Design review of the part shown in the three views and the two pictorial views. Dimensions are in mm from the part's minimum x, y and z. A direction names the side the tool comes from. Give positions to 0.01 mm unless a question says otherwise; leave off trailing zeros. Loops run counter-clockwise (first coordinate to the right, second up) from the corner with the lowest first, then second, coordinate; pieces in that order, holes last.
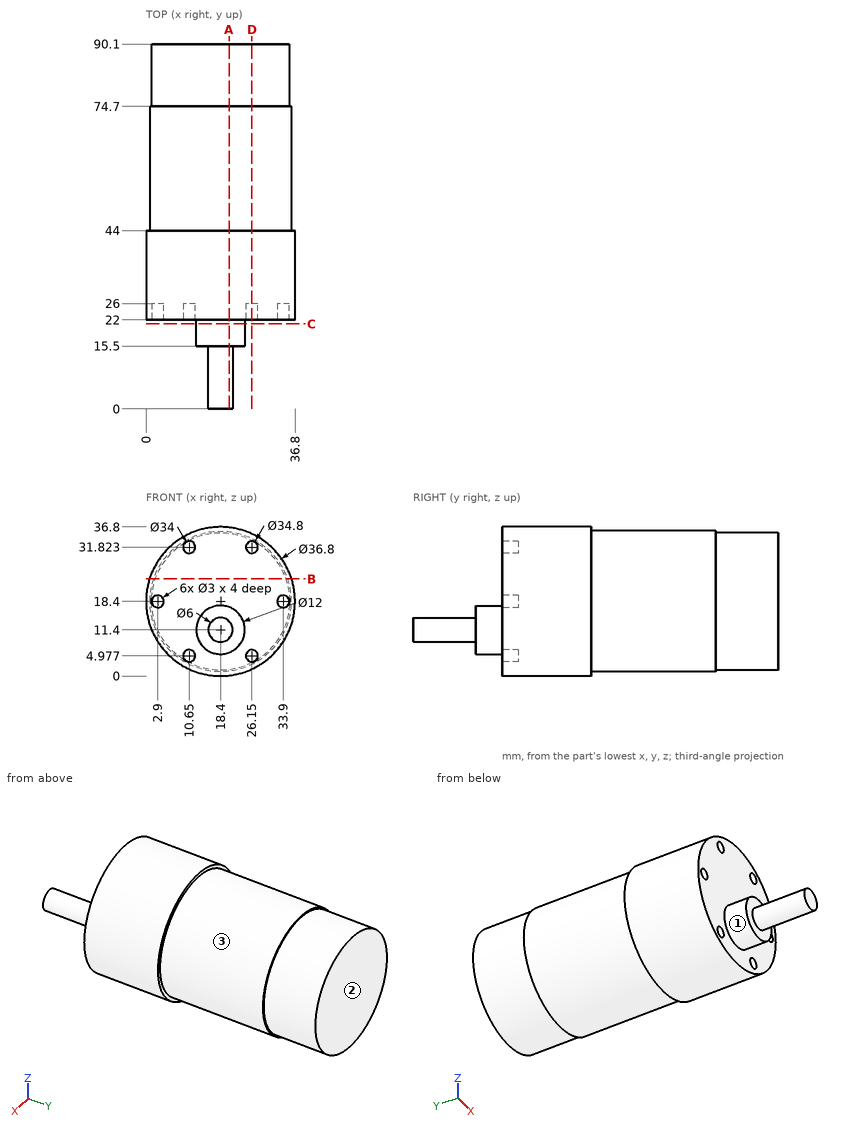
Q1. Consider section C-C on y = 21. Give the boundary of the cut face in (x, z).
Answers:
outline: circle Ø12 at (18.4, 11.4)
Q2. Consider section D-D on x = 26.15. Give the boundary of the cut face in (y, z).
Answers:
outline: (22, 1.71) - (44, 1.71) - (44, 2.82) - (74.7, 2.82) - (74.7, 3.27) - (90.1, 3.27) - (90.1, 33.53) - (74.7, 33.53) - (74.7, 33.98) - (44, 33.98) - (44, 35.09) - (22, 35.09) - (22, 33.32) - (26, 33.32) - (26, 30.32) - (22, 30.32) - (22, 6.48) - (26, 6.48) - (26, 3.48) - (22, 3.48) - close
Q3. For probe 1 along Z at (x, y) = (10.65, 23.7); probe 2 along Y at (x, z) = (15, 28.5); probe 3 along Y at (x, z) = (21, 13), list the stretches that pass through material, from the lowest coordinate up.
Answers:
probe 1: z = 1.71 to 3.48, 6.48 to 30.32, 33.32 to 35.09
probe 2: y = 22 to 90.1
probe 3: y = 15.5 to 90.1
Q4. Consider section A-A on x = 20.5. Give the boundary of the cut face in (y, z), plus the area to 3 significant figures.
Answers:
outline: (0, 9.26) - (15.5, 9.26) - (15.5, 5.78) - (22, 5.78) - (22, 0.12) - (44, 0.12) - (44, 1.13) - (74.7, 1.13) - (74.7, 1.53) - (90.1, 1.53) - (90.1, 35.27) - (74.7, 35.27) - (74.7, 35.67) - (44, 35.67) - (44, 36.68) - (22, 36.68) - (22, 17.02) - (15.5, 17.02) - (15.5, 13.54) - (0, 13.54) - close
area: 2,520 mm2
Q5. Machinability: for the marked faces 1, 2 and 3, which of the approach directions +Z, -Z, +X, -X, +Y, -Y give a long, thin tool a straight path to every point of the face, cutting with its end or side? Answer none if there is none.
Answers:
face 1: -Y
face 2: +Z, -Z, +X, -X, +Y
face 3: +Y
Q6. Consider section B-B on z = 24. Give the boundary of the cut face in (x, y) (1 decimal).
Answers:
outline: (0.9, 22) - (35.9, 22) - (35.9, 44) - (34.9, 44) - (34.9, 74.7) - (34.5, 74.7) - (34.5, 90.1) - (2.3, 90.1) - (2.3, 74.7) - (1.9, 74.7) - (1.9, 44) - (0.9, 44) - close
Q7. For pin 1 Ø0.9 at (x, z) = (26.5, 5.5) entering from -Y; pin 2 Ø12 at (x, y) = (26, 47.5) entering from -Z; pin 3 Ø10 at (x, y) = (33, 43) entering from +Z, all flat-tipped, find the tip position at first contact; note any pin that passes through.
Answers:
pin 1: stops at y = 26
pin 2: stops at z = 0.2
pin 3: stops at z = 34.1
